from build123d import *

# Parameters (mm, degrees)
F0_R     = 88.9
F1_DEPTH = 3.175


with BuildPart() as f1:
    # F0 (on Right) → F1 (new body)
    with BuildSketch(Plane.YZ):
        with BuildLine():
            Line((640.988467, 558.8), (640.988181, 635))
            ThreePointArc((640.988181, 635), (589.190891, 765.909542), (461.639941, 825.5))
            Line((461.639941, 825.5), (-395.486476, 825.5))
            ThreePointArc((-395.486476, 825.5), (-533.366758, 771.456223), (-590.911533, 635))
            Line((-590.911533, 635), (-590.911533, 558.8))
            Line((-590.911533, 558.8), (-463.911533, 0))
            Line((-463.911533, 0), (513.988467, 0))
            Line((513.988467, 0), (640.988467, 558.8))
        make_face()
        with BuildLine():
            ThreePointArc((-251.186533, 700.2947), (-222.611533, 728.8697), (-194.036533, 700.2947))
            Line((-194.036533, 700.2947), (-194.036533, 90.480119))
            ThreePointArc((-194.036533, 90.480119), (-222.611533, 61.905119), (-251.186533, 90.480119))
            Line((-251.186533, 90.480119), (-251.186533, 700.2947))
        make_face(mode=Mode.SUBTRACT)
        with BuildLine():
            ThreePointArc((-168.636533, 700.328295), (-140.061533, 728.903295), (-111.486533, 700.328295))
            Line((-111.486533, 700.328295), (-111.486533, 90.513714))
            ThreePointArc((-111.486533, 90.513714), (-140.061533, 61.938714), (-168.636533, 90.513714))
            Line((-168.636533, 90.513714), (-168.636533, 700.328295))
        make_face(mode=Mode.SUBTRACT)
        with BuildLine():
            ThreePointArc((-86.086533, 700.2947), (-57.511533, 728.8697), (-28.936533, 700.2947))
            Line((-28.936533, 700.2947), (-28.936533, 90.480119))
            ThreePointArc((-28.936533, 90.480119), (-57.511533, 61.905119), (-86.086533, 90.480119))
            Line((-86.086533, 90.480119), (-86.086533, 700.2947))
        make_face(mode=Mode.SUBTRACT)
        with BuildLine():
            ThreePointArc((-3.536533, 700.2947), (25.038467, 728.8697), (53.613467, 700.2947))
            Line((53.613467, 700.2947), (53.613467, 90.480119))
            ThreePointArc((53.613467, 90.480119), (25.038467, 61.905119), (-3.536533, 90.480119))
            Line((-3.536533, 90.480119), (-3.536533, 700.2947))
        make_face(mode=Mode.SUBTRACT)
        with BuildLine():
            ThreePointArc((79.013467, 700.261105), (107.588467, 728.836105), (136.163467, 700.261105))
            Line((136.163467, 700.261105), (136.163467, 90.446524))
            ThreePointArc((136.163467, 90.446524), (107.588467, 61.871524), (79.013467, 90.446524))
            Line((79.013467, 90.446524), (79.013467, 700.261105))
        make_face(mode=Mode.SUBTRACT)
        with BuildLine():
            ThreePointArc((161.563467, 700.2947), (190.138467, 728.8697), (218.713467, 700.2947))
            Line((218.713467, 700.2947), (218.713467, 90.480119))
            ThreePointArc((218.713467, 90.480119), (190.138467, 61.905119), (161.563467, 90.480119))
            Line((161.563467, 90.480119), (161.563467, 700.2947))
        make_face(mode=Mode.SUBTRACT)
        with BuildLine():
            ThreePointArc((244.113467, 700.261105), (272.778674, 728.655262), (301.263467, 700.080119))
            Line((301.263467, 700.080119), (301.263467, 90.480119))
            ThreePointArc((301.263467, 90.480119), (272.705255, 61.905114), (244.113467, 90.446524))
            Line((244.113467, 90.446524), (244.113467, 700.261105))
        make_face(mode=Mode.SUBTRACT)
        with Locations((-400.349473, 635)):
            Circle(F0_R, mode=Mode.SUBTRACT)
        with Locations((450.488461, 635.326673)):
            Circle(F0_R, mode=Mode.SUBTRACT)
    extrude(amount=F1_DEPTH)


solid = f1.part
Can you work these out from the model? Positions are in its coordinate system, mm. A direction names the side the tool comes from. Coordinates: 2 decimals unless noted, no trailing zeros. Write each loop counter-clockwise with the first axis right and the second up, starting at its lowest first coordinate (ties: lowest second). Pieces come first, ordered by that corner, then holes.
Q1. Which directions (+Z, -Z, +X, -X, +Y, -Y) give clear straight access to the entire face, cutting with the end or side of a thin tool? Please do faces 4 (the face through (0, 153, 419)), 5 (the face through (1.565, -140.69, 728.896)).
Results found:
face 4: +Z, -Z, -X, +Y, -Y
face 5: +X, -X
Q2. Imagine slicing it at B-B, the plane y = -424. List the corners of the cut face in (x, z) for me (3 decimals), plus the area to 3 significant figures.
Results found:
outline: (0, 0) - (3.175, 0) - (3.175, 549.304) - (0, 549.304) - close; (0, 720.696) - (3.175, 720.696) - (3.175, 824.089) - (0, 824.089) - close
area: 2,070 mm2
Q3. Imagine slicing it at A-A, the plane z = 165.5. Count the separate pieces of the cut face and the enclosed holes in it, plus the area to 3 significant figures.
Results found:
separate pieces: 8
enclosed holes: 0
area: 2,070 mm2
Q4. If we mould it in two halves opening along Y, with no side actions, what happens to faces 1 (the face through (1.57, -528.3, 283.31)), 2 (the face through (1.57, 272.15, 728.65)), 3 (the face through (3.175, 153, 419))? For each: +Y half, -Y half, draft (parallel to the pull), parting line (faces both ways), or undercut.
Results found:
face 1: -Y half
face 2: undercut
face 3: draft
Q5. Please list where these lines run through material, in increasing order: L1, parallel to Z at x = 0.8, y = -139.5; L2, parallel to Z at x = 1.7, y = 308.5; L3, parallel to Z at x = 2.25, y = 277.
Results found:
L1: z = 0 to 61.94, 728.9 to 825.5
L2: z = 0 to 825.5
L3: z = 0 to 62.23, 728.33 to 825.5
Q6. For P1, Ø1.6, axis at x = 1, z = 411, coming from the -Y side; P2, Ø1, axis at x = 1, z = 413, coming from the -Y side; P3, Ø1, axis at x = 1, z = 491.5, coming from the +Y side, each with a flat end and sliding along its axis, tell me the tip position at first contact or that it passes through.
Results found:
P1: stops at y = -557.5
P2: stops at y = -557.89
P3: stops at y = 625.81
